For this review, take the finished solid that the model builds, in its own axes (mm). A direction names the side the tool comes from. Coordinates: 2 decimals unless noted, no trailing zeros. Order: outer loops, then holes, each group sorted by start corner. A loop starts at its lowest first (then second) coordinate and runs counter-clockwise, first axis right, second up. Notation, with made-up numbers: M 78,37.25 L 127,37.25 A25 ccw 127,60.25 Z; hole C 41,-35 d7. An arc over 180 degrees is marked long. Use CSV: the item, a comma, the result in double quotes.
Autodesk Inventor part; units mm, degrees
ref_plane "YZ Plane" through (0, 0, 0) normal (1, 0, 0) x (0, 1, 0)
ref_plane "XZ Plane" through (0, 0, 0) normal (0, 1, 0) x (-1, 0, 0)
ref_plane "XY Plane" through (0, 0, 0) normal (0, 0, 1) x (1, 0, 0)
sketch "Sketch1" plane through (0, 0, 0) normal (0, 1, 0) x (-1, 0, 0)
  circle A0 centre (0, 0) radius 6.5
  line L0 (7.76, 1.75) -> (6.26, 1.75)
  line L1 (6.26, 1.75) -> (6.26, -1.75)
  line L2 (6.26, -1.75) -> (7.76, -1.75)
  line L3 (7.76, -1.75) -> (7.76, 1.75)
  dimension "d0" = 13
  dimension "d8" = 1.5
  dimension "d9" = 3.5
extrude "Extrusion1" add sketch "Sketch1" along normal blind 17
sketch "Sketch2" plane through (0, 0, 0) normal (0, -1, 0) x (0, 0, -1)
  circle A0 centre (0, 0) radius 10
  dimension "d3" = 20
extrude "Extrusion2" add sketch "Sketch2" along normal blind 1.5
sketch "Sketch4" plane through (0, 17, 0) normal (0, 1, 0) x (1, 0, 0)
  circle A0 centre (0, 0) radius 6
  arc A1 (-6.26, -1.75) -> (-6.26, 1.75) centre (0, 0) ccw
  line L0 (4.1533, 5) -> (-4.1533, 5)
  point P0 (3.3166, 5)
  point P1 (-3.3166, 5)
  dimension "d10" = 12
  dimension "d27" = 5
extrude "Extrusion3" add sketch "Sketch4" along normal blind 6 contours A0 L0 picked at (-0.7721, -1.8319)
sketch "Sketch5" plane through (0, 23, 0) normal (0, 1, 0) x (1, 0, 0)
  point P0 (0, 0)
  point P1 (0, 0)
hole "Hole1" at (0, 23, 0) direction (0, -1, 0) diameter 3.4 depth 9 tip angle 118
sketch "Sketch6" plane through (0, 0, 0) normal (0, 0, 1) x (1, 0, 0)
  circle A0 centre (0, 20) radius 1
  line L0 (6, 23) -> (-6, 23)
  line L1 (0, -4.6) -> (0, 27.6)
  point P0 (0, 0)
  dimension "d21" = 2
  dimension "d26" = 3
extrude "Extrusion4" cut sketch "Sketch6" against normal up to surface
properties part number "wheel_adapt"
Item 1: Add section C-C on y = 20. State the section outline as (x, z) points, and give its area (3 significant figures).
Solutions:
outline,"M -3.32,-5 L -1,-5 L -1,-1.37 A1.7 cw long 1,-1.37 L 1,-5 L 3.32,-5 A6 ccw long Z"
area,"92.7 mm^2"
Item 2: Add section A-A on y = 15.5. State the section outline as (x, z) points.
Solutions:
outline,"M -7.76,-1.75 L -6.26,-1.75 A6.5 ccw long -6.26,1.75 L -7.76,1.75 Z; hole C 0,0 d3.4"
Item 3: To check wall thickness, follow line 1 along Z through (x, y) = (0, 16.75); line 2 along X through (y, z) = (19.25, 0); line 3 along Y through (x, z) = (0, -2.25). State the ranges of each line that lie inside material, in increasing order. Write a range as [from, to].
Solutions:
line 1,"[-6.5, -1.7], [1.7, 6.5]"
line 2,"[-6, -1.7], [1.7, 6]"
line 3,"[-1.5, 19], [21, 23]"
Item 4: Add section D-D on z = 2.5. State the section outline as (x, y) points, and give its area (4 significant figures).
Solutions:
outline,"M -9.68,-1.5 L 9.68,-1.5 L 9.68,0 L 6,0 L 6,17 L 5.45,17 L 5.45,23 L -5.45,23 L -5.45,17 L -6,17 L -6,0 L -9.68,0 Z"
area,"298.5 mm^2"
Item 5: For faces 4 (the face through (-0.6, 17, -5.3)), 5 (the face through (-7, 8, 1.75)), 6 (the face through (-7.76, 8, 0)), list the 3-axis set-ups (+Z, -Z, +X, -X, +Y, -Y) from which the entire face can be reached by the end or side of a thin tool; tool diameter is ignored.
Solutions:
face 4,"+Y"
face 5,"+Z, -X, +Y"
face 6,"+Z, -Z, -X, +Y"
Item 6: Add section B-B on z = 4.5. State the section outline as (x, y) points, and give its area (3 significant figures).
Solutions:
outline,"M -8.93,-1.5 L 8.93,-1.5 L 8.93,0 L 4.69,0 L 4.69,17 L 3.97,17 L 3.97,23 L -3.97,23 L -3.97,17 L -4.69,17 L -4.69,0 L -8.93,0 Z"
area,"234 mm^2"
Item 7: Clearance check with flat-ended pins moving along their axes: pin 1 Ø5 at (x, y) = (3.5, 15.5) entering from +Z; pin 2 Ø1 at (y, z) = (14.5, -4) entering from +X; pin 3 Ø6 at (y, z) = (6, -0.5) entering from +X. State where each tip first meets the part, or that it passes through.
Solutions:
pin 1,"z = 6.42"
pin 2,"x = 5.48"
pin 3,"x = 6.5"
Item 8: Draft analysis for pull direction Z (two halves, no side actions). For faces 1 (the face through (6.495, 8.381, -0.261)), 2 (the face through (-0.288, 13.156, -0.064)), 3 (the face through (1, 21, -5)), state which applies: released by +Z, released by -Z, zero draft, split by the parting line, or undercut.
Solutions:
face 1,"split by the parting line"
face 2,"undercut"
face 3,"released by -Z"
